from build123d import *

# Parameters (mm, degrees)
F0_R     = 20.354373
F1_DEPTH = 60.96
F2_R     = 5.08
F3_W     = 19.056432
F3_H     = 31.234418
F4_DEPTH = 16.256


with BuildPart() as f1:
    # F0 (on Top) → F1 (new body)
    with BuildSketch(Plane.XY):
        with BuildLine():
            Line((61.058927, -14.842805), (61.058927, 40.159032))
            Line((61.058927, 40.159032), (-61.058927, 40.159032))
            ThreePointArc((-61.058927, 40.159032), (-101.217959, 0), (-61.058927, -40.159032))
            Line((-61.058927, -40.159032), (38.626283, -40.159032))
            ThreePointArc((38.626283, -40.159032), (54.111335, -31.283429), (61.058927, -14.842805))
        make_face()
        with Locations((-40.952704, 3.168637)):
            Circle(F0_R, mode=Mode.SUBTRACT)
    extrude(amount=F1_DEPTH)

    # F2
    f2_edges = [f1.edges().sort_by_distance(p)[0] for p in [
        (61.058927, 40.159032, 30.48),
    ]]
    fillet(f2_edges, radius=F2_R)

    # F3 (on face) → F4 (join)
    with BuildSketch(Plane.XY.offset(60.96)):
        with Locations((30.708643, 0)):
            Rectangle(F3_W, F3_H)
    extrude(amount=F4_DEPTH)


solid = f1.part
Geometry check sheet. Reference: the model listing, model coordinates, mm. A direction names the side the tool comes from. Round coordinates to 2 decimals unless told otherwise and drop trailing zeros. Write each loop counter-clockwise with the first axis right and the second up, starting at its lowest first coordinate (ties: lowest second). Pieces come first, ordered by that corner, then holes. Notation, with made-up numbers: (-3.5, 17.25) - (41.5, 17.25) arc R10 ccw to (41.5, 22.25) - close; hole circle Ø4 at (46, 71). An arc over 180 degrees is marked (long way). One line per item, written item: value.
1. Cross-section at A-A on y = 8. Record the boundary of the cut face in (x, z), and give its area (3 significant figures).
The answers:
outline: (-100.41, 0) - (-60.73, 0) - (-60.73, 60.96) - (-100.41, 60.96) - close; (-21.18, 0) - (61.06, 0) - (61.06, 60.96) - (40.24, 60.96) - (40.24, 77.22) - (21.18, 77.22) - (21.18, 60.96) - (-21.18, 60.96) - close
area: 7,740 mm^2
2. Cross-section at C-C on z = 34. Record the boundary of the cut face in (x, y).
The answers:
outline: (-61.06, -40.16) - (38.63, -40.16) arc R27.93 ccw to (61.06, -14.84) - (61.06, 35.08) arc R5.08 ccw to (55.98, 40.16) - (-61.06, 40.16) arc R40.16 ccw to start; hole circle Ø40.71 at (-40.95, 3.17)
3. Mould release check, pull along Y, two halves, no side actions. Record for faces 1 (the face through (-2, 40.159, 30)), 2 (the face through (-21.538, 9.283, 30.053)), 3 (the face through (-101.21, 0.88, 30.05)), 4 (the face through (-21, 9, 60.96)): released by +Y, released by -Y, zero draft, split by the parting line, or undercut.
The answers:
face 1: released by +Y
face 2: undercut
face 3: split by the parting line
face 4: zero draft
4. Scan lines: L1, parallel to Y at x = -42, z = 30.5; L2, parallel to Z at x = 47, y = 4; L3, parallel to X at y = 12, z = 31.5. Record each from-to range of solid material in increasing order.
The answers:
L1: y = -40.16 to -17.16, 23.5 to 40.16
L2: z = 0 to 60.96
L3: x = -99.38 to -59.29, -22.61 to 61.06
5. Depth check by flat-ended pin: pin 1 Ø18 at (x, z) = (33.5, 73) entering from -Y; pin 2 Ø1.5 at (x, y) = (-4.5, -6) entering from -Z; pin 3 Ø8 at (x, z) = (34, 70.5) entering from +Y; pin 4 Ø1 at (x, y) = (12, -11) entering from +Z. Enter the tip coordinate at first touch or a pass-through.
The answers:
pin 1: stops at y = -15.62
pin 2: stops at z = 0
pin 3: stops at y = 15.62
pin 4: stops at z = 60.96
6. Set-up check for faces 5 (the face through (40.237, 0, 69)), 6 (the face through (31, -15.617, 69)), 7 (the face through (61.059, 10, 30)), 8 (the face through (21.18, 0, 69)), 9 (the face through (31, 15.617, 69)): record each of +Z, -Z, +X, -X, +Y, -Y from which the full face is reachable in a straight line by a thin tool's end or side.
The answers:
face 5: +Z, +X, +Y, -Y
face 6: +Z, +X, -X, -Y
face 7: +Z, -Z, +X, +Y, -Y
face 8: +Z, -X, +Y, -Y
face 9: +Z, +X, -X, +Y
7. Cross-section at B-B on x = -44.5. Record the boundary of the cut face in (y, z), and give its area (3 significant figures).
The answers:
outline: (-40.16, 0) - (-16.87, 0) - (-16.87, 60.96) - (-40.16, 60.96) - close; (23.21, 0) - (40.16, 0) - (40.16, 60.96) - (23.21, 60.96) - close
area: 2,450 mm^2
8. Cross-section at D-D on y = -5. Record the boundary of the cut face in (x, z).
The answers:
outline: (-100.91, 0) - (-59.6, 0) - (-59.6, 60.96) - (-100.91, 60.96) - close; (-22.31, 0) - (61.06, 0) - (61.06, 60.96) - (40.24, 60.96) - (40.24, 77.22) - (21.18, 77.22) - (21.18, 60.96) - (-22.31, 60.96) - close
